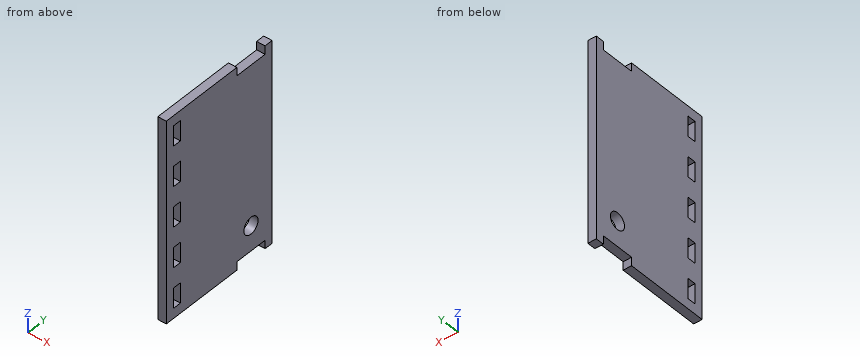
from build123d import *

# Parameters (mm, degrees)
SKETCH1_R           = 3.175
SKETCH1_W           = 7.62
SKETCH1_H           = 3.175
BOSS_EXTRUDE1_DEPTH = 1.5875


with BuildPart() as part:
    # Sketch1 → Boss-Extrude1 (new body, symmetric)
    with BuildSketch(Plane(origin=(0, 0, 0), x_dir=(0, 0, -1), z_dir=(1, 0, 0))):
        Polygon((-38.1, -23.8125), (38.1, -23.8125), (38.1, 7.9375), (34.925, 7.9375), (34.925, 20.6375), (38.1, 20.6375), (38.1, 23.8125), (-38.1, 23.8125), (-38.1, 20.6375), (-34.925, 20.6375), (-34.925, 7.9375), (-38.1, 7.9375), align=None)
        with Locations((25.4, 14.2875)):
            Circle(SKETCH1_R, mode=Mode.SUBTRACT)
        with Locations((-15.24, -19.05)):
            Rectangle(SKETCH1_W, SKETCH1_H, mode=Mode.SUBTRACT)
        with Locations((-30.48, -19.05)):
            Rectangle(SKETCH1_W, SKETCH1_H, mode=Mode.SUBTRACT)
        with Locations((0, -19.05)):
            Rectangle(SKETCH1_W, SKETCH1_H, mode=Mode.SUBTRACT)
        with Locations((15.24, -19.05)):
            Rectangle(SKETCH1_W, SKETCH1_H, mode=Mode.SUBTRACT)
        with Locations((30.48, -19.05)):
            Rectangle(SKETCH1_W, SKETCH1_H, mode=Mode.SUBTRACT)
    extrude(amount=BOSS_EXTRUDE1_DEPTH, both=True)


solid = part.part
Could you check a few things on this model? Use its own coordinates, in mm. Give positions to 0.01 mm unless a question says otherwise; leave off trailing zeros. Order: outer loops, then holes, each group sorted by start corner. A loop starts at its lowest first (then second) coordinate and runs counter-clockwise, first axis right, second up.
Item 1: I need wall thicknesses on line 1 (Z direction, x = 0.85, y = -19); line 2 (Y direction, x = -0.45, z = -25.4); line 3 (Y direction, x = 0.05, z = 18.5). Which ranges of each line are inside material? Lowest first, please.
Item 2: If we section it at C-C, the plane z = 2: Write out the boundary of the cut face in (x, y).
Item 3: I'm going to push flat-ended pins straight in: pin 1 (4 mm diameter, centred on y = 14.29, z = -25.4, fed in from -X); pin 2 (1.6 mm diameter, centred on x = 0.5, y = 12.5, fed in from -Z) (3 decimals). Where does each tip first touch, or does it pass through?
Item 4: If we section it at B-B, the plane x = -0.1: Count the separate pieces of the cut face and the enclosed holes in it, plus the area to 3 significant figures.
Item 5: If we section it at A-A, the plane z = -25.4: Write out the boundary of the cut face in (x, y).
Values:
1. line 1: z = -38.1 to -34.29, -26.67 to -19.05, -11.43 to -3.81, 3.81 to 11.43, 19.05 to 26.67, 34.29 to 38.1
1. line 2: y = -23.81 to 11.11, 17.46 to 23.81
1. line 3: y = -23.81 to -20.64, -17.46 to 23.81
2. outline: (-1.59, -23.81) - (1.59, -23.81) - (1.59, -20.64) - (-1.59, -20.64) - close; (-1.59, -17.46) - (1.59, -17.46) - (1.59, 23.81) - (-1.59, 23.81) - close
3. pin 1: passes through
3. pin 2: stops at z = -34.925
4. separate pieces: 1
4. enclosed holes: 6
4. area: 3,400 mm2
5. outline: (-1.59, -23.81) - (1.59, -23.81) - (1.59, 11.11) - (-1.59, 11.11) - close; (-1.59, 17.46) - (1.59, 17.46) - (1.59, 23.81) - (-1.59, 23.81) - close
